Read the model definition and answer for the solid it produces. Units are mm, in the model's axes. A direction names the side the tool comes from. Give positions to 0.01 mm unless a question says otherwise; leave off trailing zeros. Write each loop counter-clockwise with the first axis right and the second up, starting at its lowest first coordinate (ties: lowest second). Pieces come first, ordered by that corner, then holes. Notation, with made-up numbers: M 41,31 L 56,31 A9 ccw 56,47 Z; hole C 39.25,67 d1. An arc over 180 degrees is marked long. Use a Markdown table: item, result. Add a question column.
Item 1: A cutting plane is placed at A-A on x = -10. Determine the outline of the cut face in (y, z).
Item 2: A cutting plane is placed at D-D on x = 9. Determine the outline of the cut face in (y, z).
Item 3: Given P1, Ø0.9, axis at y = 8, z = 1, coming from the +X side; P2, Ø3, axis at x = 3, y = 2, coming from the -Z side; P3, Ø5, axis at x = 0.5, z = 1, coming from the +Y side; P4, Ø4, axis at x = -1.5, y = 4.5, coming from the +Z side, each flat-ended and moving along its own axis, determine where each tip first touches the part or whether it passes through.
Item 4: The mould has two halves that part along X. Classify faces 3 (the cylindrical face through (-12.932, 2.588, 5.362)), 4 (the flat face through (5, 8, 0)), 5 (the flat face through (5.3, 5.25, 11.5)), 6 (the cylindrical face through (-6.19, 4.44, -7.75)): pulls with the +X half, pulls with the -X half, needs draft (parallel to the pull), parting line crosses it, or undercut.
Item 5: Consider probe 1 along X at (y, z) = (7.75, 9); probe 2 along Z at (x, y) = (0, 2.5) (3 decimals); probe 3 along Z at (x, y) = (-5, 5.5). Determine where each line is inside the solid, lowest interval first. Write a range as [from, to].
Item 6: A cutting plane is placed at C-C on y = 7.5. Determine the outline of the cut face in (x, z).
Item 7: For faces 1 (the cylindrical face through (-5.325, 4.436, 10.125)), 2 (the flat face through (-2.3, 6.75, 2.5)), determine the directions among +Z, -Z, +X, -X, +Y, -Y from which every point of the face is accessible in a straight line to the end or side of a thin tool.
Item 8: A cutting plane is placed at B-B on z = 8. Determine the outline of the cut face in (x, y), then the cut area to 3 significant figures.
Autodesk Inventor part; units mm, degrees
ref_plane "YZ Plane" through (0, 0, 0) normal (1, 0, 0) x (0, 1, 0)
ref_plane "XZ Plane" through (0, 0, 0) normal (0, 1, 0) x (-1, 0, 0)
ref_plane "XY Plane" through (0, 0, 0) normal (0, 0, 1) x (1, 0, 0)
sketch "Sketch1" plane through (0, 0, 0) normal (0, 1, 0) x (-1, 0, 0)
  circle A0 centre (0, 0) radius 14
  dimension "d0" = 28
extrude "Extrusion1" add sketch "Sketch1" along normal blind 5.25
sketch "Sketch2" plane through (0, 5.25, 0) normal (0, 1, 0) x (1, 0, 0)
  circle A0 centre (0, 0) radius 12.5
  dimension "d3" = 25
extrude "Extrusion2" add sketch "Sketch2" along normal blind 3.5
sketch "Sketch3" plane through (0, 8.75, 0) normal (0, 1, 0) x (1, 0, 0)
  circle A0 centre (-10, 0) radius 1.5
  circle A1 centre (-5, -8.6603) radius 1.5
  circle A2 centre (5, -8.6603) radius 1.5
  circle A3 centre (10, 0) radius 1.5
  circle A4 centre (5, 8.6603) radius 1.5
  circle A5 centre (-5, 8.6603) radius 1.5
  arc A6 (-10, -4) -> (-10, 4) centre (-10, 0) ccw
  line L0 (-10, 4) -> (-11.8427, 4)
  circle A7 centre (0, 0) radius 12.5
  line L1 (-10, -4) -> (-11.8427, -4)
  circle A8 centre (-5, -8.6603) radius 1.5
  arc A9 (-1.5359, -10.6603) -> (-8.4641, -6.6603) centre (-5, -8.6603) ccw
  line L2 (-8.4641, -6.6603) -> (-9.3855, -8.2561)
  line L3 (-1.5359, -10.6603) -> (-2.4573, -12.2561)
  circle A10 centre (5, -8.6603) radius 1.5
  arc A11 (8.4641, -6.6603) -> (1.5359, -10.6603) centre (5, -8.6603) ccw
  line L4 (1.5359, -10.6603) -> (2.4573, -12.2561)
  line L5 (8.4641, -6.6603) -> (9.3855, -8.2561)
  circle A12 centre (10, 0) radius 1.5
  arc A13 (10, 4) -> (10, -4) centre (10, 0) ccw
  line L6 (10, -4) -> (11.8427, -4)
  line L7 (10, 4) -> (11.8427, 4)
  circle A14 centre (5, 8.6603) radius 1.5
  arc A15 (1.5359, 10.6603) -> (8.4641, 6.6603) centre (5, 8.6603) ccw
  line L8 (8.4641, 6.6603) -> (9.3855, 8.2561)
  line L9 (1.5359, 10.6603) -> (2.4573, 12.2561)
  circle A16 centre (-5, 8.6603) radius 1.5
  arc A17 (-8.4641, 6.6603) -> (-1.5359, 10.6603) centre (-5, 8.6603) ccw
  line L10 (-1.5359, 10.6603) -> (-2.4573, 12.2561)
  line L11 (-8.4641, 6.6603) -> (-9.3855, 8.2561)
  dimension "d10" = 360
  dimension "d15" = 8
  dimension "d18" = 360
extrude "Extrusion3" cut sketch "Sketch3" against normal through all contours A0 | A1 | A2 | A3 | A4 | A5
sketch "Sketch4" plane through (0, 8.75, 0) normal (0, 1, 0) x (1, 0, 0)
  line L0 (0, -5.7735) -> (-5, -2.8868)
  line L1 (-5, -2.8868) -> (-5, 2.8868)
  line L2 (-5, 2.8868) -> (0, 5.7735)
  line L3 (0, 5.7735) -> (5, 2.8868)
  line L4 (5, 2.8868) -> (5, -2.8868)
  line L5 (5, -2.8868) -> (0, -5.7735)
  point P0 (0, 0)
  point P1 (0, 0)
  dimension "d22" = 5
extrude "Extrusion4" cut sketch "Sketch4" against normal blind 2
sketch "Sketch5" plane through (0, 0, 0) normal (0, -1, 0) x (1, 0, 0)
  circle A0 centre (0, 0) radius 2.125
  dimension "d28" = 4.25
extrude "Extrusion5" cut sketch "Sketch5" against normal through all
chamfer "Chamfer2" distance 0.25 angle 45 6 edges at (2.5, 8.75, 4.3301) (5, 8.75, 0) (2.5, 8.75, -4.3301) (-2.5, 8.75, -4.3301) (-5, 8.75, 0) (-2.5, 8.75, 4.3301)
sketch "Sketch6" plane through (0, 6.75, 0) normal (0, 1, 0) x (1, 0, 0)
  circle A0 centre (0, 0) radius 3
  dimension "d34" = 6
extrude "Extrusion6" cut sketch "Sketch6" against normal blind 0.5
properties part number "Shaft_Joint1" material "ABS Plastic"
Filled in:
| question | item | result |
|---|---|---|
| 1 | outline | M 0,-9.8 L 5.25,-9.8 L 5.25,-7.5 L 8.75,-7.5 L 8.75,-1.5 L 0,-1.5 Z; M 0,1.5 L 8.75,1.5 L 8.75,7.5 L 5.25,7.5 L 5.25,9.8 L 0,9.8 Z |
| 2 | outline | M 0,-10.72 L 5.25,-10.72 L 5.25,-8.67 L 8.75,-8.67 L 8.75,-1.12 L 0,-1.12 Z; M 0,1.12 L 8.75,1.12 L 8.75,8.67 L 5.25,8.67 L 5.25,10.72 L 0,10.72 Z |
| 3 | P1 | x = 12.49 |
| 3 | P2 | z = -13.92 |
| 3 | P3 | y = 6.75 |
| 3 | P4 | z = 14 |
| 4 | face 3 | parting line crosses it |
| 4 | face 4 | undercut |
| 4 | face 5 | needs draft |
| 4 | face 6 | undercut |
| 5 | probe 1 | [-8.67, -6.46], [-3.54, 3.54], [6.46, 8.67] |
| 5 | probe 2 | [-14, -2.125], [2.125, 14] |
| 5 | probe 3 | [-11.46, -10.16], [-7.16, 7.16], [10.16, 11.46] |
| 6 | outline | C 0,0 d25; hole C -10,0 d3; hole C -5,-8.66 d3; hole C -5,8.66 d3; hole M -5,-2.89 L 0,-5.77 L 5,-2.89 L 5,2.89 L 0,5.77 L -5,2.89 Z; hole C 5,-8.66 d3; hole C 5,8.66 d3; hole C 10,0 d3 |
| 7 | face 1 | +Y, -Y |
| 7 | face 2 | +Y |
| 8 | outline | M -11.49,0 L -6.35,0 L -6.35,8.75 L -9.6,8.75 L -9.6,5.25 L -11.49,5.25 Z; M -3.65,0 L 3.65,0 L 3.65,8.75 L -3.65,8.75 Z; M 6.35,0 L 11.49,0 L 11.49,5.25 L 9.6,5.25 L 9.6,8.75 L 6.35,8.75 Z |
| 8 | area | 141 mm² |
